Model file for the job. Use its own axes, mm. A direction names the side the tool comes from. Give positions to 0.01 mm unless a question says otherwise; leave off trailing zeros. Loops run counter-clockwise (first coordinate to the right, second up) from the corner with the lowest first, then second, coordinate; pieces in that order, holes last. Notation, with made-up numbers: (80.25, 8) -> (86.25, 8) arc R18 cw to (86.25, 18) -> close; hole circle Ø1 at (40, 9.5). An arc over 180 degrees is marked (long way). Use CSV: the item, a comma, the result in double quotes. Start each with the question number.
(1) 3-axis set-ups, long thin cutter, end or side, ignore diameter. For faces 4 (the flat face through (3.131, 5.525, 15.831)), 5 (the flat face through (-3, -5, 12.7)): which of +Z, -Z, +X, -X, +Y, -Y reach the whole face in a straight line?
(2) Cut at D-D on x = -5. Write the cut outline in (y, z), then the cut area to 3 significant figures.
(3) Cut at B-B on z = 15.5. Write the cut outline in (x, y) (3 decimals).
(4) Pull direction X, two halves, no side cores. Call faces 1 (the flat face through (-3, -2, 19.05)), 2 (the cylindrical face through (-0.69, -3.1, 9.66)), 3 (the flat face through (6.35, 0, 16)): pulls with the +X half, pulls with the -X half, needs draft (parallel to the pull), parting line crosses it, or undercut.
(5) Cut at C-C on x = 2.5. Write the cut outline in (y, z).
(6) Flat gauge pins, fed straight in: pin 1 (3 mm diameter, centred on y = -5.5, z = 7.5, fed in from +X); pin 2 (1 mm diameter, centred on x = 4, z = 9, fed in from -Y). Where does each tip first touch, or does it go through?
(7) Drill centre lines: probe 1 along Y at (x, z) = (0, 6.5) (1 decimal); probe 2 along Y at (x, z) = (-2.5, 8.5); probe 3 along X at (y, z) = (1.75, 13.5). Where is each one in solid material? Low to high.
Autodesk Inventor part; units mm, degrees
ref_plane "YZ Plane" through (0, 0, 0) normal (1, 0, 0) x (0, 1, 0)
ref_plane "XZ Plane" through (0, 0, 0) normal (0, 1, 0) x (-1, 0, 0)
ref_plane "XY Plane" through (0, 0, 0) normal (0, 0, 1) x (1, 0, 0)
sketch "Sketch1" plane through (0, 0, 0) normal (0, 0, 1) x (1, 0, 0)
  circle A0 centre (0, 0) radius 5.3975
  dimension "d0" = 10.795
extrude "Extrusion1" add sketch "Sketch1" along normal blind 12.7
thread "Thread1"
sketch "Sketch2" plane through (0, 0, 12.7) normal (0, 0, 1) x (1, 0, 0)
  circle A0 centre (0, 0) radius 5.3975
  line L0 (0, 7.3323) -> (6.35, 3.6662)
  line L1 (6.35, 3.6662) -> (6.35, -3.6662)
  line L2 (6.35, -3.6662) -> (0, -7.3323)
  line L3 (0, -7.3323) -> (-6.35, -3.6662)
  line L4 (-6.35, -3.6662) -> (-6.35, 3.6662)
  line L5 (-6.35, 3.6662) -> (0, 7.3323)
  dimension "d5" = 12.7
  dimension "d6" = 0
extrude "Extrusion2" add sketch "Sketch2" along normal blind 6.35 contours A0 | L0 L1 L2 L3 L4 L5
sketch "Sketch5" plane through (0, 0, 19.05) normal (0, 0, 1) x (1, 0, 0)
  circle A0 centre (0, 0) radius 3.175
  dimension "d14" = 6.35
extrude "Extrusion5" cut sketch "Sketch5" against normal through all
properties part number "Pnematic Screw Part 1764"
Check result:
1,face 4,"+Z, -Z, +X, +Y"
1,face 5,"-Z"
2,outline,"(-4.45, 12.7) -> (-2.03, 12.7) -> (-2.03, 0) -> (2.03, 0) -> (2.03, 12.7) -> (4.45, 12.7) -> (4.45, 19.05) -> (-4.45, 19.05) -> close"
2,area,"108 mm²"
3,outline,"(-6.35, -3.666) -> (0, -7.332) -> (6.35, -3.666) -> (6.35, 3.666) -> (0, 7.332) -> (-6.35, 3.666) -> close; hole circle Ø6.35 at (0, 0)"
4,face 1,"needs draft"
4,face 2,"undercut"
4,face 3,"pulls with the +X half"
5,outline,"(-5.89, 12.7) -> (-4.78, 12.7) -> (-4.78, 0) -> (-1.96, 0) -> (-1.96, 19.05) -> (-5.89, 19.05) -> close; (1.96, 0) -> (4.78, 0) -> (4.78, 12.7) -> (5.89, 12.7) -> (5.89, 19.05) -> (1.96, 19.05) -> close"
6,pin 1,"x = 3.62"
6,pin 2,"y = -4.11"
7,probe 1,"-5.4 to -3.2, 3.2 to 5.4"
7,probe 2,"-4.78 to -1.96, 1.96 to 4.78"
7,probe 3,"-6.35 to -2.65, 2.65 to 6.35"
